Input: part model. Units: mm. Frame: model coordinates. Face numbers are marked on the shaded views. A direction names the side the tool comes from. Round coordinates to 2 decimals unless told otherwise and drop trailing zeros. Order: outer loops, then holes, each group sorted by start corner. A loop starts at its lowest first (then second) coordinate and runs counter-clockwise, first axis right, second up.
Item 1: Cut plane B-B on x = -5.25. Output: boundary loops of the cut face in (y, z), then the cut area to 3 significant figures.
Item 2: Line query: L1, parallel to Z at x = -3.75, y = -1.15; L2, parallel to Z at x = 1.5, y = -1.5; L3, parallel to X at y = -0.4, z = 2.75. Output: solid intervals per line, ascending.
Item 3: First-contact query: pin 1 (2 mm diameter, centred on y = -0.5, z = 4.5, fed in from +X); pin 2 (0.7 mm diameter, centred on y = 1.5, z = -1.5, fed in from -X); pin 3 (0.7 mm diameter, centred on x = -5.5, y = -1.5, fed in from +Z). Flat tips, straight axial feed; report the tip coordinate or a pass-through.
Item 4: Reachability of the marked faces 1 and 2 from +Z, -Z, +X, -X, +Y, -Y: full face, straight path, thin tool, end or side. Return the list, or none.
Item 5: Cut plane A-A on z = -1. Output: boundary loops of the cut face in (x, y).
Item 6: Mould query, pull axis Y, two halves, no side actions, for the marked faces 3, 4, 5 and 6. Classes: released by +Y, released by -Y, zero draft, split by the parting line, or undercut.
Item 7: Cut plane D-D on x = -1.75. Output: boundary loops of the cut face in (y, z).
Item 8: Cut plane C-C on y = 0. Output: boundary loops of the cut face in (x, z), then the cut area to 3 significant figures.
```python
from build123d import *

# Parameters (mm, degrees)
SKETCH3_W           = 0.64
SKETCH3_H           = 0.64
BOSS_EXTRUDE1_DEPTH = 2.683
ESQUISSE1_W         = 0.64
ESQUISSE1_H         = 0.64
BOSS_EXTRU_1_DEPTH  = 10
CONG_1_R            = 1
CONG_1_2_R          = 0.5


with BuildPart() as part:
    # Sketch2 → Base-Revolve (revolve)
    with BuildSketch(Plane(origin=(0, 0, 0), x_dir=(0, 0, -1), z_dir=(1, 0, 0))):
        with BuildLine():
            Line((0, 0), (0, 2.55))
            Line((0, 2.55), (-1, 2.55))
            Line((-1, 2.55), (-1, 2.05))
            Line((-1, 2.05), (-6.55, 2.05))
            ThreePointArc((-6.55, 2.05), (-7.999568901, 1.449568901), (-8.6, 0))
            Line((-8.6, 0), (0, 0))
        make_face()
    revolve(axis=Axis((0, 0, 0), (0, 0, 1)))

    # Sketch3 → Boss-Extrude1 (add)
    with BuildSketch(Plane(origin=(0, 0, 0), x_dir=(-1, 0, 0), z_dir=(0, 0, -1))):
        with Locations((0, 1.27)):
            Rectangle(SKETCH3_W, SKETCH3_H)
        with Locations((0, -1.27)):
            Rectangle(SKETCH3_W, SKETCH3_H)
    extrude(amount=BOSS_EXTRUDE1_DEPTH)

    # Esquisse1 → Boss.-Extru.1 (add)
    with BuildSketch(Plane(origin=(0.32, 0, 0), x_dir=(0, 0, -1), z_dir=(1, 0, 0))):
        with Locations((2.683, -1.27)):
            Rectangle(ESQUISSE1_W, ESQUISSE1_H)
        with Locations((2.683, 1.27)):
            Rectangle(ESQUISSE1_W, ESQUISSE1_H)
    extrude(amount=-BOSS_EXTRU_1_DEPTH)

    # Cong_1
    cong_1_edges = [part.edges().sort_by_distance(p)[0] for p in [
        (0.32, -1.27, -3.003),
        (0.32, 1.27, -3.003),
    ]]
    fillet(cong_1_edges, radius=CONG_1_R)

    # Cong_1 2
    cong_1_2_edges = [part.edges().sort_by_distance(p)[0] for p in [
        (-0.32, 1.27, -2.363),
        (-0.32, -1.27, -2.363),
    ]]
    fillet(cong_1_2_edges, radius=CONG_1_2_R)


solid = part.part
```
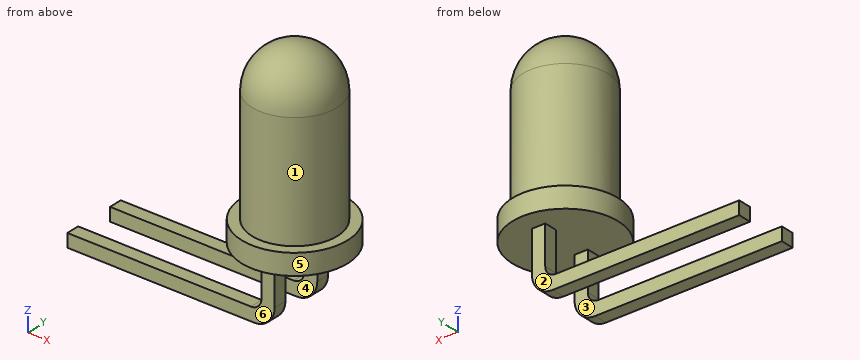
From the geometry:
1. outline: (-1.59, -3) - (-0.95, -3) - (-0.95, -2.36) - (-1.59, -2.36) - close; (0.95, -3) - (1.59, -3) - (1.59, -2.36) - (0.95, -2.36) - close
1. area: 0.819 mm2
2. L1: z = -3 to -2.36
2. L2: z = 0 to 1
2. L3: x = -2.01 to 2.01
3. pin 1: stops at x = 2.05
3. pin 2: stops at x = -0.32
3. pin 3: stops at z = -2.36
4. face 1: +Z
4. face 2: -Z, +X, -X, +Y
5. outline: (-0.32, -1.59) - (0.32, -1.59) - (0.32, -0.95) - (-0.32, -0.95) - close; (-0.32, 0.95) - (0.32, 0.95) - (0.32, 1.59) - (-0.32, 1.59) - close
6. face 3: undercut
6. face 4: undercut
6. face 5: split by the parting line
6. face 6: released by -Y
7. outline: (-1.85, 0) - (1.85, 0) - (1.85, 1) - (1.07, 1) - (1.07, 6.55) arc R1.07 ccw to (-1.07, 6.55) - (-1.07, 1) - (-1.85, 1) - close; (-1.59, -3) - (-0.95, -3) - (-0.95, -2.36) - (-1.59, -2.36) - close; (0.95, -3) - (1.59, -3) - (1.59, -2.36) - (0.95, -2.36) - close
8. outline: (-2.55, 0) - (2.55, 0) - (2.55, 1) - (2.05, 1) - (2.05, 6.55) arc R2.05 ccw to (-2.05, 6.55) - (-2.05, 1) - (-2.55, 1) - close
8. area: 34.5 mm2
